Could you check a few things on this model? Use its own coordinates, in mm. A direction names the side the tool comes from. Give positions to 0.01 mm unless a question says otherwise; leave off trailing zeros. Order: outer loops, then holes, each group sorted by start corner. A loop starts at its lowest first (then second) coordinate and runs counter-clockwise, first axis right, second up. Notation, with made-up numbers: M -14,49.25 L 12,49.25 A14 cw 12,68.25 Z; hole C 31.25,-10 d3. An arc over 180 degrees is marked long. Answer in a Markdown table with one row per item. Add a question column.
```python
from build123d import *

# Parameters (mm, degrees)
F1_DEPTH  = 42
F3_DEPTH  = 112.001
F2_R      = 9.5
F4_DEPTH  = 112.001
F6_DEPTH  = 3
F8_DEPTH  = 22
F10_DEPTH = 19.001


with BuildPart() as f1:
    # F0 (on Front) → F1 (new body)
    with BuildSketch(Plane.XZ):
        Polygon((-133, 0), (0, 0), (0, 16), (-21, 16), (-21, 66), (-43, 66), (-43, 16), (-133, 16), align=None)
    extrude(amount=F1_DEPTH)

    # F2 (on face) → F3 (cut, through all)
    with BuildSketch(Plane.YZ.offset(-21)):
        with BuildLine():
            Line((-42, 66), (-42, 44.820994))
            ThreePointArc((-42, 44.820994), (-21, 65.820994), (0, 44.820994))
            Line((0, 44.820994), (0, 66))
            Line((0, 66), (-42, 66))
        make_face()
    extrude(amount=-F3_DEPTH, mode=Mode.SUBTRACT)

    # F2 (on face) → F4 (cut, through all)
    with BuildSketch(Plane.YZ.offset(-21)):
        with Locations((-21, 44.820994)):
            Circle(F2_R)
    extrude(amount=-F4_DEPTH, mode=Mode.SUBTRACT)

    # F5 (on face) → F6 (join)
    with BuildSketch(Plane.XY.offset(16)):
        with BuildLine():
            Line((-64, -8), (-108, -8))
            ThreePointArc((-108, -8), (-121, -21), (-108, -34))
            Line((-108, -34), (-64, -34))
            ThreePointArc((-64, -34), (-51, -21), (-64, -8))
        make_face()
    extrude(amount=F6_DEPTH)

    # F7 (on Front) → F8 (join)
    with BuildSketch(Plane.XZ):
        with BuildLine():
            Line((-130, 0), (-9, 0))
            ThreePointArc((-9, 0), (-13.122975, 31.317104), (-25.210926, 60.5))
            Line((-25.210926, 60.5), (-130, 0))
        make_face()
    extrude(amount=-F8_DEPTH)

    # F9 (on face) → F10 (cut, through all)
    with BuildSketch(Plane.XY.offset(19)):
        with BuildLine():
            Line((-64, -13.062797), (-108, -13.062797))
            ThreePointArc((-108, -13.062797), (-114.5, -19.562797), (-108, -26.062797))
            Line((-108, -26.062797), (-64, -26.062797))
            ThreePointArc((-64, -26.062797), (-57.5, -19.562797), (-64, -13.062797))
        make_face()
    extrude(amount=-F10_DEPTH, mode=Mode.SUBTRACT)


solid = f1.part
```
1. Suppose I cut it at A-A on y = -15.5. List the corners of the cut face in (x, z) for me.
2. Thinking about a two-plate mould opening in X: for faces 1 (the flat face through (-76.872, 10.846, 30.673)), 2 (the flat face through (-86, -27, 19)), 3 (the cylindrical face through (-57.5, -19.7, 9.6)), 4 (the cylindrical face through (-51, -21, 17)), which applies, pulls with the +X half, pulls with the -X half, needs draft (parallel to the pull), parting line crosses it, or undercut?
3. For faces 5 (the flat face through (-86, -34, 17)), 6 (the flat face through (-86, -13.063, 10)), 7 (the cylindrical face through (-121, -21, 17)), 8 (the flat face through (-21, -21, 35)), which set-ups out of +Z, -Z, +X, -X, +Y, -Y let a thin tool reach every point of the face, with its end or its side?
4. Will these pins go through, and if not, where does the flat tip stop? P1, Ø12.5, axis at x = -77, y = -21.5, coming from the +Z side; P2, Ø4, axis at x = -69, z = 25, coming from the -Y side; P3, Ø3, axis at x = -97, y = -24, coming from the -Z side; P4, Ø6.5, axis at x = -12, y = -14.5, coming from the +Z side.
5. If I drill on line 1 along Z through (x, y) = (-32.5, -21); line 2 along Y through (x, z) = (-93.5, 10.5); line 3 along Z through (x, y) = (-105, -37.5), over which ranges is the centre line in solid material (lowest first)? Write a range as [from, to].
6. Suppose I cut it at B-B on z = 50.5. List the corners of the cut face in (x, y) for me, plus the area to 3 significant figures.
7. Suppose I cut it at C-C on x = -97. List the corners of the cut face in (y, z) for me, plus the area to 3 significant figures.
8. Suppose I cut it at D-D on z = 6. List the corners of the cut face in (x, y) for me.
Findings below:
| question | item | result |
|---|---|---|
| 1 | outline | M -133,0 L -113.07,0 L -113.07,19 L -119.78,19 L -119.78,16 L -133,16 Z; M -58.93,0 L 0,0 L 0,16 L -21,16 L -21,37.08 L -43,37.08 L -43,16 L -52.22,16 L -52.22,19 L -58.93,19 Z; M -43,52.57 L -21,52.57 L -21,65.09 L -43,65.09 Z |
| 2 | face 1 | pulls with the -X half |
| 2 | face 2 | needs draft |
| 2 | face 3 | undercut |
| 2 | face 4 | undercut |
| 3 | face 5 | +Z, -X, -Y |
| 3 | face 6 | +Z, -Z |
| 3 | face 7 | +Z, -X |
| 3 | face 8 | +Z, +X, -Y |
| 4 | P1 | z = 19 |
| 4 | P2 | y = 0 |
| 4 | P3 | through |
| 4 | P4 | z = 16 |
| 5 | line 1 | [0, 35.32], [54.32, 65.82] |
| 5 | line 2 | [-42, -26.06], [-13.06, 22] |
| 5 | line 3 | [0, 16] |
| 6 | outline | M -43,-41.22 L -21,-41.22 L -21,-28.62 L -43,-28.62 Z; M -43,-13.38 L -21,-13.38 L -21,-0.78 L -43,-0.78 Z; M -42.53,0 L -20.04,0 L -20.04,22 L -42.53,22 Z |
| 6 | area | 1,050 mm2 |
| 7 | outline | M -42,0 L -26.06,0 L -26.06,19 L -34,19 L -34,16 L -42,16 Z; M -13.06,0 L 22,0 L 22,19.05 L 0,19.05 L 0,16 L -8,16 L -8,19 L -13.06,19 Z |
| 7 | area | 922 mm2 |
| 8 | outline | M -133,-42 L 0,-42 L 0,0 L -9.15,0 L -9.15,22 L -119.61,22 L -119.61,0 L -133,0 Z; hole M -108,-26.06 L -64,-26.06 A6.5 ccw -64,-13.06 L -108,-13.06 A6.5 ccw Z |
